Here's how the part is built. I have some questions about the finished solid (model axes, mm). Round coordinates to 2 decimals unless told otherwise and drop trailing zeros. Write each loop counter-clockwise with the first axis right and the second up, starting at its lowest first coordinate (ties: lowest second). Pieces come first, ordered by that corner, then holes. Notation, with made-up numbers: (78.25, 1) - (99.25, 1) arc R17 cw to (99.25, 17) - close; hole circle Ø9 at (35.5, 81.25). An arc over 180 degrees is marked (long way). One line per item, written item: value. Start each with the question number.
Item 1: Thinking about a two-plate mould opening in Z: for faces 1 (the face through (-2, 3.175, -2)), 2 (the face through (109.225, 1.61, -127.223)), which applies, released by +Z, released by -Z, zero draft, split by the parting line, or undercut?
Item 2: If I drill on line 1 (Z direction, x = 114.3, y = 1.2); line 2 (X direction, y = 2.45, z = -127); line 3 (X direction, y = 1.45, z = -76.2), over which ranges is the centre line in solid material (lowest first)?
Item 3: Imagine slicing it at A-A, the plane y = 1.4. Please give me the cut outline in (x, z).
Item 4: For P1, Ø1, axis at y = 2, z = 19.5, coming from the +X side; P2, Ø1.6, axis at y = 1.5, z = 12.5, coming from the -X side; P3, Ø2.5, axis at x = 63.5, z = -127, coming from the -Y side, each with a flat end and sliding along its axis, tell me the tip position at first contact or that it passes through.
Item 5: Imagine slicing it at B-B, the plane z = 35.5. Please give me the cut outline in (x, y) (1 decimal).
```python
from build123d import *

# Parameters (mm, degrees)
SKETCH1_W           = 457.2
SKETCH1_H           = 279.4
BOSS_EXTRUDE1_DEPTH = 3.175
SKETCH2_R           = 5.08
CUT_EXTRUDE1_DEPTH  = 3.175
SKETCH4_R           = 2.25
CUT_EXTRUDE3_DEPTH  = 25.4
SKETCH6_R           = 2.25
CUT_EXTRUDE5_DEPTH  = 637.032
SKETCH7_R           = 5.08
SKETCH7_R_2         = 2.25
SKETCH7_W           = 1.5875
SKETCH7_H           = 31.75
CUT_EXTRUDE6_DEPTH  = 25.4


with BuildPart() as part:
    # Sketch1 → Boss-Extrude1 (new body)
    with BuildSketch(Plane(origin=(0, 0, 0), x_dir=(1, 0, 0), z_dir=(0, 1, 0))):
        Rectangle(SKETCH1_W, SKETCH1_H)
    extrude(amount=BOSS_EXTRUDE1_DEPTH)

    # Sketch2 → Cut-Extrude1 (cut)
    with BuildSketch(Plane(origin=(0, 3.175, 0), x_dir=(1, 0, 0), z_dir=(0, 1, 0))):
        with Locations((-114.3, 127)):
            Circle(SKETCH2_R)
        with Locations((114.3, 127)):
            Circle(SKETCH2_R)
        with Locations((-215.9, -127)):
            Circle(SKETCH2_R)
        with Locations((215.9, -127)):
            Circle(SKETCH2_R)
        with BuildLine():
            Line((-212.307897552, 130.592102448), (-205.957897552, 124.242102448))
            ThreePointArc((-205.957897552, 124.242102448), (-205.957897552, 117.057897552), (-213.142102448, 117.057897552))
            Line((-213.142102448, 117.057897552), (-219.492102448, 123.407897552))
            ThreePointArc((-219.492102448, 123.407897552), (-219.492102448, 130.592102448), (-212.307897552, 130.592102448))
        make_face()
        with BuildLine():
            Line((212.307897552, 130.592102448), (205.957897552, 124.242102448))
            ThreePointArc((205.957897552, 124.242102448), (205.957897552, 117.057897552), (213.142102448, 117.057897552))
            Line((213.142102448, 117.057897552), (219.492102448, 123.407897552))
            ThreePointArc((219.492102448, 123.407897552), (219.492102448, 130.592102448), (212.307897552, 130.592102448))
        make_face()
    extrude(amount=-CUT_EXTRUDE1_DEPTH, mode=Mode.SUBTRACT)

    # Sketch4 → Cut-Extrude3 (cut)
    with BuildSketch(Plane(origin=(0, 3.175, 0), x_dir=(1, 0, 0), z_dir=(0, 1, 0))):
        with Locations((-196.85, 127)):
            Circle(SKETCH4_R)
        with Locations((-215.9, 107.95)):
            Circle(SKETCH4_R)
        with Locations((196.85, 127)):
            Circle(SKETCH4_R)
        with Locations((215.9, 107.95)):
            Circle(SKETCH4_R)
    extrude(amount=-CUT_EXTRUDE3_DEPTH, mode=Mode.SUBTRACT)

    # Sketch6 → Cut-Extrude5 (cut)
    with BuildSketch(Plane(origin=(0, 3.175, 0), x_dir=(1, 0, 0), z_dir=(0, 1, 0))):
        with Locations((-215.9, 76.2)):
            Circle(SKETCH6_R)
        with Locations((-215.9, 0)):
            Circle(SKETCH6_R)
        with Locations((-215.9, -88.9)):
            Circle(SKETCH6_R)
        with Locations((-114.3, -76.2)):
            Circle(SKETCH6_R)
        with Locations((-114.3, 76.2)):
            Circle(SKETCH6_R)
        with Locations((-63.5, 127)):
            Circle(SKETCH6_R)
        with Locations((63.5, 127)):
            Circle(SKETCH6_R)
        with Locations((114.3, 76.2)):
            Circle(SKETCH6_R)
        with Locations((215.9, -88.9)):
            Circle(SKETCH6_R)
        with Locations((215.9, 0)):
            Circle(SKETCH6_R)
        with Locations((215.9, 76.2)):
            Circle(SKETCH6_R)
    extrude(amount=-CUT_EXTRUDE5_DEPTH, mode=Mode.SUBTRACT)

    # Sketch7 → Cut-Extrude6 (cut)
    with BuildSketch(Plane(origin=(0, 3.175, 0), x_dir=(1, 0, 0), z_dir=(0, 1, 0))):
        Polygon((-104.775, -44.45), (-104.775, 44.45), (-123.825, 44.45), (-123.825, 107.95), (-123.825, 139.7), (-228.6, 139.7), (-228.6, -139.7), (-123.825, -139.7), (-123.825, -107.95), (-123.825, -44.45), align=None)
        with Locations((-215.9, -127)):
            Circle(SKETCH7_R, mode=Mode.SUBTRACT)
        with Locations((-215.9, -88.9)):
            Circle(SKETCH7_R_2, mode=Mode.SUBTRACT)
        with Locations((-215.9, 0)):
            Circle(SKETCH7_R_2, mode=Mode.SUBTRACT)
        with Locations((-114.3, -19.05)):
            Circle(SKETCH7_R_2, mode=Mode.SUBTRACT)
        with Locations((-114.3, 19.05)):
            Circle(SKETCH7_R_2, mode=Mode.SUBTRACT)
        with Locations((-215.9, 76.2)):
            Circle(SKETCH7_R_2, mode=Mode.SUBTRACT)
        with Locations((-215.9, 107.95)):
            Circle(SKETCH7_R_2, mode=Mode.SUBTRACT)
        with BuildLine():
            Line((-213.142102448, 117.057897552), (-219.492102448, 123.407897552))
            ThreePointArc((-219.492102448, 123.407897552), (-219.492102448, 130.592102448), (-212.307897552, 130.592102448))
            Line((-212.307897552, 130.592102448), (-205.957897552, 124.242102448))
            ThreePointArc((-205.957897552, 124.242102448), (-205.957897552, 117.057897552), (-213.142102448, 117.057897552))
        make_face(mode=Mode.SUBTRACT)
        with Locations((-196.85, 127)):
            Circle(SKETCH7_R_2, mode=Mode.SUBTRACT)
        Polygon((228.6, 139.7), (122.2375, 139.7), (122.2375, 107.95), (122.2375, 46.0375), (103.1875, 46.0375), (103.1875, -46.0375), (122.2375, -46.0375), (122.2375, -107.95), (122.2375, -139.7), (228.6, -139.7), align=None)
        with Locations((215.9, -127)):
            Circle(SKETCH7_R, mode=Mode.SUBTRACT)
        with Locations((215.9, -88.9)):
            Circle(SKETCH7_R_2, mode=Mode.SUBTRACT)
        with Locations((215.9, 0)):
            Circle(SKETCH7_R_2, mode=Mode.SUBTRACT)
        with Locations((215.9, 76.2)):
            Circle(SKETCH7_R_2, mode=Mode.SUBTRACT)
        with Locations((215.9, 107.95)):
            Circle(SKETCH7_R_2, mode=Mode.SUBTRACT)
        with Locations((196.85, 127)):
            Circle(SKETCH7_R_2, mode=Mode.SUBTRACT)
        with BuildLine():
            Line((205.957897552, 124.242102448), (212.307897552, 130.592102448))
            ThreePointArc((212.307897552, 130.592102448), (219.492102448, 130.592102448), (219.492102448, 123.407897552))
            Line((219.492102448, 123.407897552), (213.142102448, 117.057897552))
            ThreePointArc((213.142102448, 117.057897552), (205.957897552, 117.057897552), (205.957897552, 124.242102448))
        make_face(mode=Mode.SUBTRACT)
        Polygon((-123.825, 44.45), (-104.775, 44.45), (-104.775, 46.0375), (-122.2375, 46.0375), (-122.2375, 107.95), (-122.2375, 139.7), (-123.825, 139.7), (-123.825, 107.95), align=None)
        Polygon((-104.775, 46.0375), (-104.775, 44.45), (-104.775, -44.45), (-104.775, -46.0375), (-103.1875, -46.0375), (-103.1875, 46.0375), align=None)
        Polygon((-104.775, -46.0375), (-104.775, -44.45), (-123.825, -44.45), (-123.825, -107.95), (-122.2375, -107.95), (-122.2375, -46.0375), align=None)
        with Locations((-123.03125, -123.825)):
            Rectangle(SKETCH7_W, SKETCH7_H)
        with Locations((-114.3, 19.05)):
            Circle(SKETCH7_R_2)
        with Locations((-114.3, -19.05)):
            Circle(SKETCH7_R_2)
    extrude(amount=-CUT_EXTRUDE6_DEPTH, mode=Mode.SUBTRACT)


solid = part.part
```
Values follow:
1. face 1: zero draft
1. face 2: undercut
2. line 1: z = -139.7 to -132.08, -121.92 to -78.45, -73.95 to -46.04, 46.04 to 139.7
2. line 2: x = -122.24 to -119.38, -109.22 to -65.75, -61.25 to 61.25, 65.75 to 109.22, 119.38 to 122.24
2. line 3: x = -122.24 to -116.55, -112.05 to 112.05, 116.55 to 122.24
3. outline: (-122.24, -139.7) - (122.24, -139.7) - (122.24, -46.04) - (103.19, -46.04) - (103.19, 46.04) - (122.24, 46.04) - (122.24, 139.7) - (-122.24, 139.7) - (-122.24, 46.04) - (-103.19, 46.04) - (-103.19, -46.04) - (-122.24, -46.04) - close; hole circle Ø10.16 at (-114.3, -127); hole circle Ø4.5 at (-114.3, -76.2); hole circle Ø4.5 at (-114.3, 76.2); hole circle Ø4.5 at (-63.5, -127); hole circle Ø4.5 at (63.5, -127); hole circle Ø10.16 at (114.3, -127); hole circle Ø4.5 at (114.3, -76.2)
4. P1: stops at x = 103.19
4. P2: stops at x = -103.19
4. P3: passes through
5. outline: (-103.2, 0) - (103.2, 0) - (103.2, 3.2) - (-103.2, 3.2) - close
